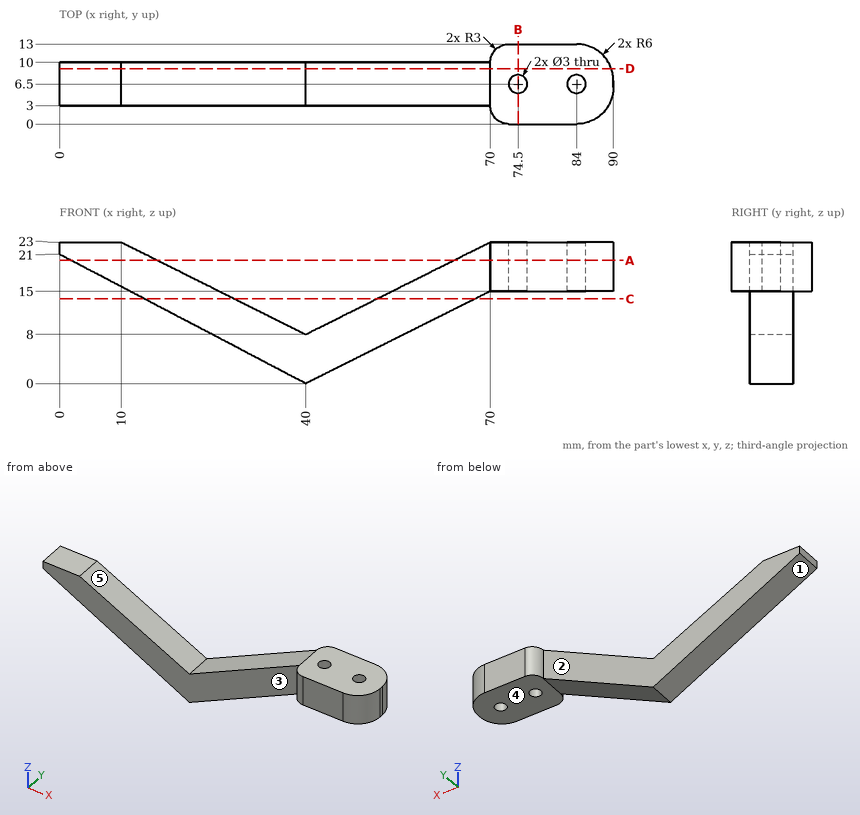
Design review of the part shown in the three views and the two pictorial views. Dimensions are in mm from the part's minimum x, y and z. A direction names the side the tool comes from. Give positions to 0.01 mm unless a question says otherwise; leave off trailing zeros. Loops run counter-clockwise (first coordinate to the right, second up) from the corner with the lowest first, then second, coordinate; pieces in that order, holes last. Notation, with made-up numbers: (38.5, -1) -> (92.5, -1) arc R29 cw to (92.5, 22) -> close; hole circle Ø4 at (43.5, 25.25). An arc over 180 degrees is marked (long way). One line per item, written item: value.
Q1. We need section B-B on x = 74.5. Give the boundary of the cut face in (y, z), and give its area (3 significant figures).
Numbers:
outline: (0, 15) -> (5, 15) -> (5, 23) -> (0, 23) -> close; (8, 15) -> (13, 15) -> (13, 23) -> (8, 23) -> close
area: 80.0 mm^2
Q2. We need section A-A on z = 20. Give the number of separate pieces and of enclosed holes in the cut face, and give its area (3 significant figures).
Numbers:
separate pieces: 2
enclosed holes: 2
area: 367 mm^2
Q3. For pin 1 Ø3.5 at (x, y) = (84, 6.5) entering from +Z; pin 2 Ø11.5 at (x, z) = (51.5, 16) entering from -Y; pin 3 Ø1.5 at (x, z) = (51.5, 10.5) entering from +Y; pin 4 Ø1.5 at (y, z) = (2, 17.5) entering from +X, all flat-tipped, find the tip position at first contact; note any pin that passes through.
Numbers:
pin 1: stops at z = 23
pin 2: stops at y = 3
pin 3: stops at y = 10
pin 4: stops at x = 89.04
Q4. Machinability: for the marked faces 1, 2, 3, 4 and 5, which of the approach directions +Z, -Z, +X, -X, +Y, -Y give a long, thin tool a straight path to every point of the face, cutting with its end or side? Answer none if there is none.
Numbers:
face 1: -Z, -X, +Y, -Y
face 2: +Z, -Z, -X, +Y
face 3: +Z, -Z, -X, -Y
face 4: -Z, +X, +Y, -Y
face 5: +Z, +Y, -Y
Q5. We need section D-D on y = 9. Give the boundary of the cut face in (x, z), and give its area (3 significant figures).
Numbers:
outline: (0, 21) -> (40, 0) -> (70, 15) -> (89.66, 15) -> (89.66, 23) -> (70, 23) -> (40, 8) -> (10, 23) -> (0, 23) -> close
area: 672 mm^2
Q6. We need section C-C on z = 13.75. Give the boundary of the cut face in (x, y), and give its area (3 significant figures).
Numbers:
outline: (13.81, 3) -> (28.5, 3) -> (28.5, 10) -> (13.81, 10) -> close; (51.5, 3) -> (67.5, 3) -> (67.5, 10) -> (51.5, 10) -> close
area: 215 mm^2
Q7. For L1, parallel to Y at x = 74.5, z = 20.5; L2, parallel to X at y = 6, z = 22.25 (1 decimal); L3, parallel to Y at x = 67, z = 14.5, list the stretches that pass through material, from the lowest coordinate up.
Numbers:
L1: y = 0 to 5, 8 to 13
L2: x = 0 to 11.5, 68.5 to 73.1, 75.9 to 82.6, 85.4 to 90
L3: y = 3 to 10
